from build123d import *

# Parameters (mm, degrees)
SKIZZE1_R                       = 14.1
AUFSATZ_LINEAR_AUSTRAGEN1_DEPTH = 15
VERRUNDUNG1_R                   = 100
SKIZZE2_R                       = 1.4
SCHNITT_LINEAR_AUSTRAGEN1_DEPTH = 10
SKIZZE3_R                       = 1.45
SCHNITT_LINEAR_AUSTRAGEN2_DEPTH = 10
SKIZZE6_R                       = 14.1
SKIZZE6_R_2                     = 12.6
AUFSATZ_LINEAR_AUSTRAGEN3_DEPTH = 1
FASE1_SIZE                      = 1
FASE2_SIZE                      = 1


with BuildPart() as part:
    # Skizze1 → Aufsatz-Linear austragen1 (new body)
    with BuildSketch(Plane.XY):
        with BuildLine():
            Line((19.722068857, 7.5), (75, 7.5))
            Line((75, 7.5), (75, -7.5))
            Line((75, -7.5), (19.722068857, -7.5))
            ThreePointArc((19.722068857, -7.5), (0, -21.1), (-19.722068857, -7.5))
            Line((-19.722068857, -7.5), (-75, -7.5))
            Line((-75, -7.5), (-75, 7.5))
            Line((-75, 7.5), (-19.722068857, 7.5))
            ThreePointArc((-19.722068857, 7.5), (0, 21.1), (19.722068857, 7.5))
        make_face()
        Circle(SKIZZE1_R, mode=Mode.SUBTRACT)
    extrude(amount=AUFSATZ_LINEAR_AUSTRAGEN1_DEPTH)

    # Verrundung1
    verrundung1_edges = [part.edges().sort_by_distance(p)[0] for p in [
        (19.722068857, -7.5, 7.5),
        (-19.722068857, -7.5, 7.5),
        (-19.722068857, 7.5, 7.5),
        (19.722068857, 7.5, 7.5),
    ]]
    fillet(verrundung1_edges, radius=VERRUNDUNG1_R)

    # Skizze2 → Schnitt-Linear austragen1 (cut)
    with BuildSketch(Plane(origin=(0, 0, 0), x_dir=(-1, 0, 0), z_dir=(0, 0, -1))):
        with Locations((-67.5, 2)):
            Circle(SKIZZE2_R)
        with Locations((67.5, 2)):
            Circle(SKIZZE2_R)
    extrude(amount=-SCHNITT_LINEAR_AUSTRAGEN1_DEPTH, mode=Mode.SUBTRACT)

    # Skizze3 → Schnitt-Linear austragen2 (cut)
    with BuildSketch(Plane(origin=(75, 0, 0), x_dir=(0, 0, -1), z_dir=(1, 0, 0))):
        with Locations((-7.5, -2)):
            Circle(SKIZZE3_R)
    schnitt_linear_austragen2 = extrude(amount=-SCHNITT_LINEAR_AUSTRAGEN2_DEPTH, mode=Mode.SUBTRACT)

    # Spiegeln1: Schnitt-Linear austragen2 across plane
    add(schnitt_linear_austragen2.mirror(Plane(origin=(0, 0, 0), x_dir=(0, 0, 1), z_dir=(1, 0, 0))), mode=Mode.SUBTRACT)

    # Skizze6 → Aufsatz-Linear austragen3 (add)
    with BuildSketch(Plane.XY.offset(15)):
        Circle(SKIZZE6_R)
        Circle(SKIZZE6_R_2, mode=Mode.SUBTRACT)
    extrude(amount=-AUFSATZ_LINEAR_AUSTRAGEN3_DEPTH)

    # Fase1
    fase1_edges = [part.edges().sort_by_distance(p)[0] for p in [
        (-14.1, 0, 0),
    ]]
    chamfer(fase1_edges, length=FASE1_SIZE)

    # Fase2
    fase2_edges = [part.edges().sort_by_distance(p)[0] for p in [
        (75, 0, 0),
        (75, -7.5, 7.5),
        (-75, -7.5, 7.5),
        (-75, 0, 0),
    ]]
    chamfer(fase2_edges, length=FASE2_SIZE)


solid = part.part
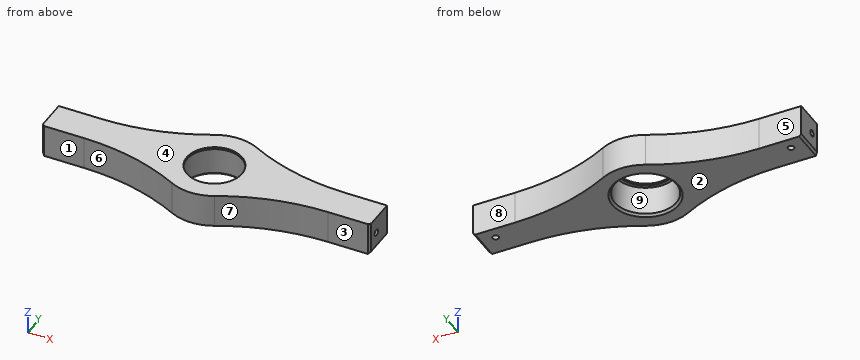
Geometry: final body of the model. Coordinates: model frame, mm. Face numbers are marked on the shaded views. A direction names the side the tool comes from. Coordinates: 2 decimals unless noted, no trailing zeros. Order: outer loops, then holes, each group sorted by start corner. A loop starts at its lowest first (then second) coordinate and runs counter-clockwise, first axis right, second up. Notation, with made-up numbers: M -21,80 L 29,80 A6 cw 29,90 Z; hole C 36.5,-14.5 d10. An arc over 180 degrees is marked long. One line per question, with ' | ' between items. Start each with the question number.
Item 1: Cut plane D-D, the plane x = 16.5. Return the cut outline in (y, z), then the cut area to 3 significant figures.
Item 2: Set-up query: the marked faces 1, 2, 3, 4 and 5. Return all of +Z, -Z, +X, -X, +Y, -Y with unobstructed straight access to the full face (end or side cutting, diameter ignored); none if empty.
Item 3: Pin query (flat end, axial travel): pin 1 Ø4.5 at (x, z) = (-69.5, 4) entering from +Y; pin 2 Ø1.5 at (x, z) = (45.5, 8) entering from +Y; pin 3 Ø5 at (x, z) = (14.5, 2) entering from -Y; pin 4 Ø15 at (x, y) = (0, 0) entering from +Z. Return the tip coordinate at first contact, or that it passes through.
Item 4: Cut plane B-B, the plane x = -67.5. Return the cut outline in (y, z).
Item 5: Draft query along X for the marked faces 6, 7, 8 and 9. Return one class per face: released by +X, released by -X, zero draft, split by the parting line, or undercut.
Item 6: Cut plane A-A, the plane z = 3. Return the cut outline in (x, y), then the cut area to 3 significant figures.
Item 7: Ray query, probe 1 along Y at (x, z) = (72.5, 7.5); probe 2 along Y at (x, z) = (67.5, 6.5); probe 3 along Y at (x, z) = (67.5, 4). Return the intervals inside material, ascending. Write a range as [from, to].
Item 8: Cut plane C-C, the plane x = 62.5. Return the cut outline in (y, z), then the cut area to 3 significant figures.
A:
1) outline: M -15.53,0 L 15.53,0 L 15.53,15 L -15.53,15 Z | area: 466 mm2
2) face 1: +Z, -Z, -X, -Y | face 2: -Z, +X, -X, +Y, -Y | face 3: +Z, -Z, +X, -Y | face 4: +Z, +X, -X, +Y, -Y | face 5: +Z, -Z, -X, +Y
3) pin 1: stops at y = 7.5 | pin 2: stops at y = 8.11 | pin 3: stops at y = -17.58 | pin 4: passes through
4) outline: M -7.5,0 L 0.6,0 L 0.6,10 L 3.4,10 L 3.4,0 L 7.5,0 L 7.5,15 L -7.5,15 Z; hole C -2,7.5 d2.9
5) face 6: released by -X | face 7: released by +X | face 8: zero draft | face 9: undercut
6) outline: M -75,-6.5 L -74,-7.5 L -55.76,-7.5 A100 cw -9.72,-18.73 A21.1 ccw 9.72,-18.73 A100 cw 55.76,-7.5 L 74,-7.5 L 75,-6.5 L 75,7.5 L 55.76,7.5 A100 cw 9.72,18.73 A21.1 ccw -9.72,18.73 A100 cw -55.76,7.5 L -75,7.5 Z; hole C -67.5,2 d2.8; hole C 0,0 d28.2; hole C 67.5,2 d2.8 | area: 2,780 mm2
7) probe 1: y = [-7.5, -3.45], [-0.55, 7.5] | probe 2: y = [-7.5, -3.05], [-0.95, 0.6], [3.4, 7.5] | probe 3: y = [-7.5, 0.6], [3.4, 7.5]
8) outline: M -7.5,0 L 7.5,0 L 7.5,15 L -7.5,15 Z | area: 225 mm2
